Answer from the drawing. Dimensions are ordinates in mm from the lowest x, y and z of the part. A direction names the side the tool comes from. Give positions to 0.01 mm unless a question says otherwise; leave off trailing zeros. Loops run counter-clockwise (first coordinate to the right, second up) from the corner with the lowest first, then second, coordinate; pieces in that order, holes last.
Item 1: Each of these flat-tipped pins is pushed along its axis until it touches: pin 1 Ø12 at (y, z) = (6.5, 3) entering from -X; pin 2 Ø8 at (x, y) = (13.5, 9.5) entering from +Z (3 decimals). Where does it stop, or does it pass through?
Item 2: Section C-C, the plane z = 12.75 is taken. Give the vertices of the cut face in (x, y) (3 decimals).
Item 3: A tool of negligible diameter and unlimited length cuts with its end or side. For the marked faces 1 and 2, from which of +Z, -Z, +X, -X, +Y, -Y can it reach the whole face along a straight path? Write none if from no direction.
Item 4: Section D-D, the plane x = 6.75 is taken. Give the vertices of the cut face in (y, z) (3 decimals).
Item 5: Section A-A, the plane x = 20 is taken. Give the vertices of the cut face in (y, z) (3 decimals).
Item 6: Consider line 1 along Y through (x, z) = (14, 18) (3 decimals); line 2 along Y through (x, z) = (2.5, 2.25). Determine where each line is inside the solid, lowest interval first.
Item 7: Section B-B, the plane y = 7.5 is taken. Give the vertices of the cut face in (x, z) (3 decimals), and give its area (3 significant figures).
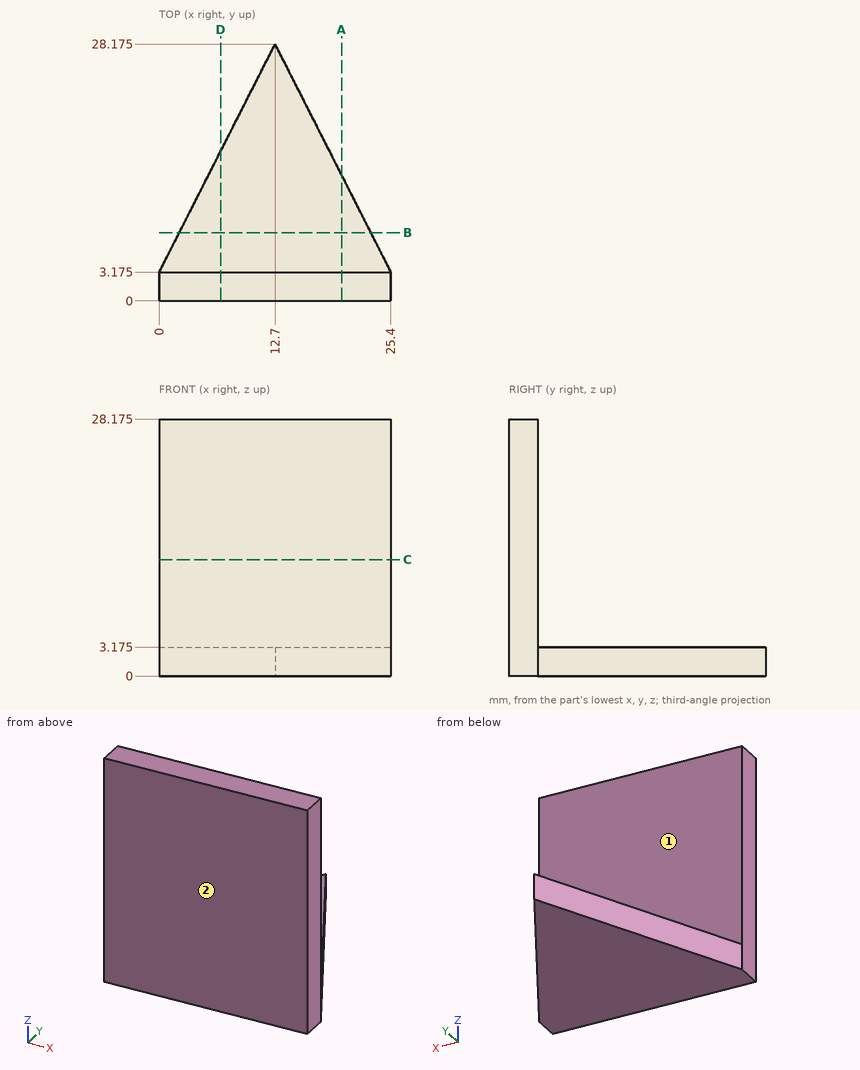
Worked answers:
1. pin 1: stops at x = 0
1. pin 2: stops at z = 3.175
2. outline: (0, 0) - (25.4, 0) - (25.4, 3.175) - (0, 3.175) - close
3. face 1: +Z, +X, -X, +Y
3. face 2: +Z, -Z, +X, -X, -Y
4. outline: (0, 0) - (16.462, 0) - (16.462, 3.175) - (3.175, 3.175) - (3.175, 28.175) - (0, 28.175) - close
5. outline: (0, 0) - (13.805, 0) - (13.805, 3.175) - (3.175, 3.175) - (3.175, 28.175) - (0, 28.175) - close
6. line 1: y = 0 to 3.175
6. line 2: y = 0 to 8.1
7. outline: (2.197, 0) - (23.203, 0) - (23.203, 3.175) - (2.197, 3.175) - close
7. area: 66.7 mm2
